```python
from build123d import *

# Parameters (mm, degrees)
SKETCH1_W           = 15.5
SKETCH1_H           = 13.5
BOSS_EXTRUDE1_DEPTH = 67
SKETCH2_W           = 7.62
SKETCH2_H           = 9.779
BOSS_EXTRUDE2_DEPTH = 5.588
SKETCH4_W           = 1.524
SKETCH4_H           = 5.842


with BuildPart() as part:
    # Sketch1 → Boss-Extrude1 (new body)
    with BuildSketch(Plane(origin=(0, 0, 0), x_dir=(0, 0, -1), z_dir=(1, 0, 0))):
        Rectangle(SKETCH1_W, SKETCH1_H)
    extrude(amount=BOSS_EXTRUDE1_DEPTH)

    # Sketch2 → Boss-Extrude2 (add)
    with BuildSketch(Plane.XY.offset(7.75)):
        with Locations((13.81, -1.8605)):
            Rectangle(SKETCH2_W, SKETCH2_H)
    extrude(amount=BOSS_EXTRUDE2_DEPTH)

    # Sweep1: sweep along a path in Sketch3
    with BuildLine(Plane(origin=(0, 0, 0), x_dir=(1, 0, 0), z_dir=(0, 1, 0))) as sweep1_path:
        Line((-0.762, 7.75), (-0.762, -7.242))
        ThreePointArc((-0.762, -7.242), (-0.390025612, -8.140025612), (0.508, -8.512))
        Line((0.508, -8.512), (10, -8.512))
    # Sketch4 → Sweep1 (sweep)
    with BuildSketch(Plane.ZY.offset(-10)):
        with Locations((9.528, -1.8605)):
            Rectangle(SKETCH4_W, SKETCH4_H)
    sweep(path=sweep1_path.line)


solid = part.part
```
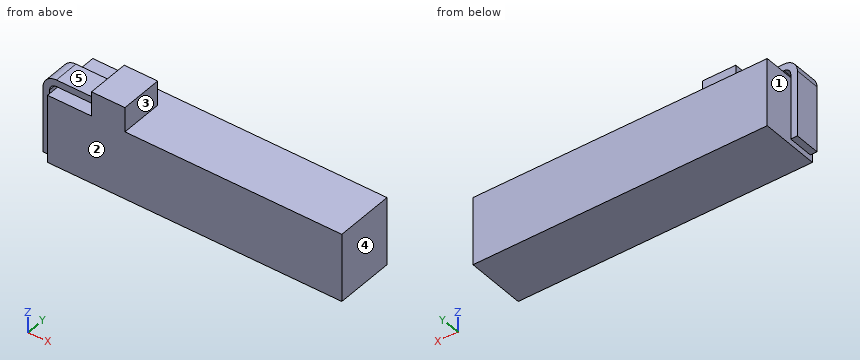
Geometry check sheet. Reference: the model listing, model coordinates, mm. Face numbers are marked on the shaded views. A direction names the side the tool comes from. Coordinates: 2 decimals unless noted, no trailing zeros. Write each loop counter-clockwise with the first axis right and the second up, starting at its lowest first coordinate (ties: lowest second). Pieces come first, ordered by that corner, then holes. Notation, with made-up numbers: M -19.75,69.25 L 31.25,69.25 A19 cw 31.25,74.25 Z; hole C -33,-25.75 d9. An arc over 180 degrees is marked long. One line per item, written item: value. Start each with the question number.
(1) Sectioned sample at B-B, the plane x = 8.5. Enter the section's corners in (y, z).
(2) Scan lines: line 1 along X through (y, z) = (1, -2.5); line 2 along Y through (x, z) = (12, 10); line 3 along Z through (x, y) = (30.5, -5). Record each from-to range of solid material in increasing order. Write a range as [from, to].
(3) Tool access check on the marked faces 1, 2, 3, 4 and 5. Record the directions out of +Z, -Z, +X, -X, +Y, -Y that give a thin tool (end or side, any length) a straight path to the whole face; none if there is none.
(4) Sectioned sample at C-C, the plane y = -4. Enter the section's corners in (x, z).
(5) Sectioned sample at A-A, the plane z = 6. Enter the section's corners in (x, y), and give its area (3 significant figures).
(6) Depth check by flat-ended pin: pin 1 (3 mm diameter, centred on x = 44, y = -1, fed in from +Z); pin 2 (1.7 mm diameter, centred on y = 0.5, z = 11.5, fed in from +X); pin 3 (1.7 mm diameter, centred on y = -4, z = 11.5, fed in from -X). Enter the tip coordinate at first touch or a pass-through.
(7) Sectioned sample at D-D, the plane x = 17. Enter the section's corners in (y, z).
Filled sheet:
1. outline: M -6.75,-7.75 L 6.75,-7.75 L 6.75,7.75 L -6.75,7.75 Z; M -4.78,8.77 L 1.06,8.77 L 1.06,10.29 L -4.78,10.29 Z
2. line 1: [-2.54, -1.02], [0, 67]
2. line 2: [-6.75, 3.03]
2. line 3: [-7.75, 7.75]
3. face 1: -Z, +Y, -Y
3. face 2: +Z, -Z, +X, -X, -Y
3. face 3: +Z, +X, +Y, -Y
3. face 4: +Z, -Z, +X, +Y, -Y
3. face 5: +Z, -X, +Y, -Y
4. outline: M -2.54,-7.75 L -1.02,-7.75 L -1.02,7.24 A1.52 cw 0.51,8.77 L 10,8.77 L 10,7.75 L 0,7.75 L 0,-7.75 L 67,-7.75 L 67,7.75 L 17.62,7.75 L 17.62,13.34 L 10,13.34 L 10,10.29 L 0.51,10.29 A3.05 ccw -2.54,7.24 Z
5. outline: M -2.54,-4.78 L -1.02,-4.78 L -1.02,1.06 L -2.54,1.06 Z; M 0,-6.75 L 67,-6.75 L 67,6.75 L 0,6.75 Z
5. area: 913 mm²
6. pin 1: z = 7.75
6. pin 2: x = 17.62
6. pin 3: x = 10
7. outline: M -6.75,-7.75 L 6.75,-7.75 L 6.75,7.75 L 3.03,7.75 L 3.03,13.34 L -6.75,13.34 Z
